```python
from build123d import *

# Parameters (mm, degrees)
ESQUISSE1_R        = 1.6
BOSS_EXTRU_1_DEPTH = 2
CHANFREIN1_SIZE    = 2


with BuildPart() as part:
    # Esquisse1 → Boss.-Extru.1 (new body)
    with BuildSketch(Plane.XY):
        with BuildLine():
            Line((-36.5, -58.3), (36.5, -58.3))
            ThreePointArc((36.5, -58.3), (39.540559159, -57.040559159), (40.8, -54))
            Line((40.8, -54), (40.8, 54))
            ThreePointArc((40.8, 54), (39.540559159, 57.040559159), (36.5, 58.3))
            Line((36.5, 58.3), (-36.5, 58.3))
            ThreePointArc((-36.5, 58.3), (-39.540559159, 57.040559159), (-40.8, 54))
            Line((-40.8, 54), (-40.8, -54))
            ThreePointArc((-40.8, -54), (-39.540559159, -57.040559159), (-36.5, -58.3))
        make_face()
        with Locations((35.93, -49.1)):
            Circle(ESQUISSE1_R, mode=Mode.SUBTRACT)
        with Locations((-35.93, -49.1)):
            Circle(ESQUISSE1_R, mode=Mode.SUBTRACT)
        with Locations((-20, 34)):
            Circle(ESQUISSE1_R, mode=Mode.SUBTRACT)
        with Locations((20, 34)):
            Circle(ESQUISSE1_R, mode=Mode.SUBTRACT)
    extrude(amount=-BOSS_EXTRU_1_DEPTH)

    # Chanfrein1
    chanfrein1_edges = [part.edges().sort_by_distance(p)[0] for p in [
        (34.33, -49.1, 0),
        (-37.53, -49.1, 0),
        (-21.6, 34, 0),
        (18.4, 34, 0),
    ]]
    chamfer(chanfrein1_edges, length=CHANFREIN1_SIZE - 0.0001)  # a hair under: the kernel refuses the full size


solid = part.part
```
The model under review builds one solid part; all positions refer to its coordinate system, in mm. Round coordinates to 2 decimals unless told otherwise and drop trailing zeros. Use CSV: the item, a comma, the result in double quotes. Start each with the question number.
(1) Clearance check with flat-ended pins moving along their axes: P1, Ø1.5, axis at x = -2, y = 38, coming from the +Z side; P2, Ø5, axis at x = -20, y = 34, coming from the +Z side; P3, Ø3.5, axis at x = -35.93, y = -49.1, coming from the +Z side. State where each tip first meets the part, or that it passes through.
(2) We need section B-B, the plane y = 34. State how many separate pieces and enclosed holes the cut face has, then the cut area to 3 significant figures.
(3) For line 1 along X through (y, z) = (34, -1.95); line 2 along X through (y, z) = (-48, -0.05); line 3 along Y through (x, z) = (21, -0.3), list the stretches that pass through material, from the lowest coordinate up.
Findings:
1,P1,"z = 0"
1,P2,"z = -1.1"
1,P3,"z = -1.85"
2,separate pieces,"3"
2,enclosed holes,"0"
2,area,"142 mm^2"
3,line 1,"-40.8 to -21.65, -18.35 to 18.35, 21.65 to 40.8"
3,line 2,"-40.8 to -39.31, -32.55 to 32.55, 39.31 to 40.8"
3,line 3,"-58.3 to 30.86, 37.14 to 58.3"
